```python
from build123d import *

# Parameters (mm, degrees)
SKETCH1_R           = 1.45
SKETCH1_R_2         = 1.6
BOSS_EXTRUDE1_DEPTH = 4
SKETCH2_R           = 4
SKETCH2_R_2         = 1.45
BOSS_EXTRUDE2_DEPTH = 3
SKETCH3_R           = 25
CUT_EXTRUDE1_DEPTH  = 10
FILLET1_R           = 5


with BuildPart() as part:
    # Sketch1 → Boss-Extrude1 (new body)
    # profile 1 of 3: a face of its own
    with BuildSketch(Plane(origin=(0, 0, 0), x_dir=(1, 0, 0), z_dir=(0, 1, 0))):
        with BuildLine():
            ThreePointArc((6, 0), (5.247620154, 2.909034672), (3.179172425, 5.088502991))
            ThreePointArc((3.179172425, 5.088502991), (-3.872509642, 4.582976007), (-5.547666284, -2.285475619))
            ThreePointArc((-5.547666284, -2.285475619), (-4.582976007, -3.872509642), (-3.179172425, -5.088502991))
            ThreePointArc((-3.179172425, -5.088502991), (2.909034672, -5.247620154), (6, 0))
        make_face()
        with Locations(Location((0, 0, 0), (0, 0, 270))):
            Circle(SKETCH1_R, mode=Mode.SUBTRACT)
    # profile 2 of 3: a face of its own
    with BuildSketch(Plane(origin=(0, 0, 0), x_dir=(1, 0, 0), z_dir=(0, 1, 0))):
        with BuildLine():
            Line((31.029172425, -12.311497009), (3.179172425, 5.088502991))
            ThreePointArc((3.179172425, 5.088502991), (5.247620154, 2.909034672), (6, 0))
            ThreePointArc((6, 0), (2.909034672, -5.247620154), (-3.179172425, -5.088502991))
            Line((-3.179172425, -5.088502991), (24.670827575, -22.488502991))
            ThreePointArc((24.670827575, -22.488502991), (22.602379846, -20.309034672), (21.85, -17.4))
            ThreePointArc((21.85, -17.4), (23.259082466, -13.536908466), (26.824492066, -11.488288448))
            ThreePointArc((26.824492066, -11.488288448), (29.002816451, -11.511790235), (31.029172425, -12.311497009))
        make_face()
    # profile 3 of 3: a face of its own
    with BuildSketch(Plane(origin=(0, 0, 0), x_dir=(1, 0, 0), z_dir=(0, 1, 0))):
        with BuildLine():
            ThreePointArc((33.85, -17.4), (33.097620154, -14.490965328), (31.029172425, -12.311497009))
            ThreePointArc((31.029172425, -12.311497009), (29.002816451, -11.511790235), (26.824492066, -11.488288448))
            ThreePointArc((26.824492066, -11.488288448), (23.259082466, -13.536908466), (21.85, -17.4))
            ThreePointArc((21.85, -17.4), (22.602379846, -20.309034672), (24.670827575, -22.488502991))
            ThreePointArc((24.670827575, -22.488502991), (30.759034672, -22.647620154), (33.85, -17.4))
        make_face()
        with Locations(Location((27.85, -17.4, 0), (0, 0, 270))):
            Circle(SKETCH1_R_2, mode=Mode.SUBTRACT)
    extrude(amount=BOSS_EXTRUDE1_DEPTH)

    # Sketch2 → Boss-Extrude2 (add)
    with BuildSketch(Plane(origin=(0, 4, 0), x_dir=(1, 0, 0), z_dir=(0, 1, 0))):
        with Locations(Location((0, 0, 0), (0, 0, 270))):
            Circle(SKETCH2_R)
        with Locations(Location((0, 0, 0), (0, 0, 270))):
            Circle(SKETCH2_R_2, mode=Mode.SUBTRACT)
    extrude(amount=BOSS_EXTRUDE2_DEPTH)

    # Sketch3 → Cut-Extrude1 (cut)
    with BuildSketch(Plane(origin=(0, 4, 0), x_dir=(1, 0, 0), z_dir=(0, 1, 0))):
        with Locations((-2.15, -30)):
            Circle(SKETCH3_R)
        with Locations((26.019288726, 15.087051209)):
            Circle(SKETCH3_R)
    extrude(amount=-CUT_EXTRUDE1_DEPTH, mode=Mode.SUBTRACT)

    # Fillet1
    fillet1_edges = [part.edges().sort_by_distance(p)[0] for p in [
        (-3.277923152, 2, 5.025457174),
        (20.790880187, 2, 20.064406598),
        (27.149225038, 2, 9.887400616),
        (3.079209508, 2, -5.149608607),
    ]]
    fillet(fillet1_edges, radius=FILLET1_R)


solid = part.part
```
Read the model definition and answer for the solid it produces. Units are mm, in the model's axes. A direction names the side the tool comes from. Give positions to 0.01 mm unless a question says otherwise; leave off trailing zeros. Order: outer loops, then holes, each group sorted by start corner. A loop starts at its lowest first (then second) coordinate and runs counter-clockwise, first axis right, second up. Notation, with made-up numbers: (12, -38) -> (52, -38) arc R31 ccw to (52, -13) -> close; hole circle Ø5 at (-33, 22.25). An arc over 180 degrees is marked (long way). Write item = value, one per line.
1. A cutting plane is placed at A-A, the plane x = 27.85. Write down the section's boundary in (y, z), and give its area (3 significant figures).
Numbers:
outline = (0, 10.37) -> (4, 10.37) -> (4, 15.8) -> (0, 15.8) -> close; (0, 19) -> (4, 19) -> (4, 23.4) -> (0, 23.4) -> close
area = 39.3 mm²
2. A cutting plane is placed at D-D, the plane y = 5. Write down the section's boundary in (x, z), and give its area (3 significant figures).
Numbers:
outline = circle Ø8 at (0, 0); hole circle Ø2.9 at (0, 0)
area = 43.7 mm²
3. A cutting plane is placed at B-B, the plane z = 18. Write down the section's boundary in (x, y).
Numbers:
outline = (19.78, 0) -> (26.37, 0) -> (26.37, 4) -> (19.78, 4) -> close; (29.33, 0) -> (33.82, 0) -> (33.82, 4) -> (29.33, 4) -> close
4. Given pin 1 (3 mm diameter, centred on x = 3, y = 3.5, fed in from +Z); pin 2 (4 mm diameter, centred on x = 15, y = 4, fed in from -Z); pin 3 (1.5 mm diameter, centred on x = 12, y = 3.5, fed in from -Z), each flat-ended and moving along its own axis, determine where each tip first touches the part or whether it passes through.
Numbers:
pin_1 = 5.9
pin_2 = 6.26
pin_3 = 5.08
5. A cutting plane is placed at C-C, the plane y = 3.25. Count the separate pieces of the cut face and the enclosed holes in it, and give its area (3 significant figures).
Numbers:
separate_pieces = 1
enclosed_holes = 2
area = 319 mm²
6. For faces 1 (the face through (0.06, 3.45, -1.45)), 2 (the face through (-3.905, 5.479, -0.867)), determine the directions among +Z, -Z, +X, -X, +Y, -Y from which every point of the face is accessible in a straight line to the end or side of a thin tool.
Numbers:
face_1 = +Y, -Y
face_2 = +Y
7. The mould has two halves that part along X. Classify faces 3 (the face through (29.73, 1.97, 11.5)), 4 (the face through (21.007, 2.028, 19.985)), 5 (the face through (28.331, 1.972, 18.926)): +X half, -X half, draft (parallel to the pull), parting line (faces both ways), or undercut.
Numbers:
face_3 = +X half
face_4 = -X half
face_5 = undercut
8. Straight lines are drawn through the part: line 1 along Y through (x, z) = (20.5, 16.25); line 2 along X through (y, z) = (2.05, 17.4); line 3 along X through (y, z) = (2.5, 0). For each, find the intervals that lie inside material, in ascending order.
Numbers:
line_1 = 0 to 4
line_2 = 19.44 to 26.25, 29.45 to 33.85
line_3 = -6 to -1.45, 1.45 to 6.08
